```python
from build123d import *

# Parameters (mm, degrees)
SKETCH1_W           = 62
SKETCH1_H           = 42
BOSS_EXTRUDE1_DEPTH = 30
SKETCH2_R           = 10
CUT_EXTRUDE1_DEPTH  = 6
CUT_EXTRUDE2_START  = -2
SKETCH3_W           = 60
SKETCH3_H           = 40
CUT_EXTRUDE2_DEPTH  = 27
CUT_EXTRUDE3_REACH  = 62.547
SKETCH4_W           = 60
SKETCH4_H           = 28
SKETCH5_W           = 20
SKETCH5_H           = 1
CUT_EXTRUDE4_DEPTH  = 27
BOSS_EXTRUDE2_START = 2
BOSS_EXTRUDE2_DEPTH = 5
BOSS_EXTRUDE3_START = -7
BOSS_EXTRUDE3_DEPTH = 5
SKETCH10_W          = 15.255500618
SKETCH10_H          = 40
CUT_EXTRUDE5_DEPTH  = 1


with BuildPart() as part:
    # Sketch1 → Boss-Extrude1 (new body)
    with BuildSketch(Plane.XY):
        with Locations((0.653781513, -2.494957983)):
            Rectangle(SKETCH1_W, SKETCH1_H)
    extrude(amount=BOSS_EXTRUDE1_DEPTH)

    # Sketch2 → Cut-Extrude1 (cut)
    with BuildSketch(Plane.XY.offset(30)):
        with Locations((-15.346218487, -8.494957983)):
            Circle(SKETCH2_R)
    extrude(amount=-CUT_EXTRUDE1_DEPTH, mode=Mode.SUBTRACT)

    # Sketch3 → Cut-Extrude2 (cut)
    with BuildSketch(Plane.XY.offset(30).offset(CUT_EXTRUDE2_START)):
        with Locations((0.653781513, -2.494957983)):
            Rectangle(SKETCH3_W, SKETCH3_H)
    extrude(amount=-CUT_EXTRUDE2_DEPTH, mode=Mode.SUBTRACT)

    # Cut-Extrude3: up to this face of the body (flat: up to its plane)
    cut_extrude3_end = Plane(part.part.faces().sort_by_distance((0.653781513, -22.494957983, 14.5))[0])
    # Sketch4 → Cut-Extrude3 (cut, up to the picked face)
    with BuildSketch(Plane(origin=(0, 18.505042017, 0), x_dir=(1, 0, 0), z_dir=(0, 1, 0)), mode=Mode.PRIVATE) as cut_extrude3_sk1:
        with Locations((0.653781513, -15)):
            Rectangle(SKETCH4_W, SKETCH4_H)
    cut_extrude3_tool1 = split(extrude(cut_extrude3_sk1.sketch, amount=-CUT_EXTRUDE3_REACH, mode=Mode.PRIVATE), bisect_by=cut_extrude3_end, keep=Keep.BOTH, mode=Mode.PRIVATE)
    add(cut_extrude3_tool1.solids().sort_by(Axis((0.653782, 18.505042, 15), (0, -1, 0)))[0], mode=Mode.SUBTRACT)

    # Sketch5 → Cut-Extrude4 (cut)
    with BuildSketch(Plane(origin=(0, 18.505042017, 0), x_dir=(1, 0, 0), z_dir=(0, 1, 0))):
        with Locations((-15.346218487, -29.5)):
            Rectangle(SKETCH5_W, SKETCH5_H)
    extrude(amount=-CUT_EXTRUDE4_DEPTH, mode=Mode.SUBTRACT)

    # Sketch7 → Boss-Extrude2 (add)
    with BuildSketch(Plane(origin=(0, 0, 0), x_dir=(0, 0, -1), z_dir=(1, 0, 0)).offset(BOSS_EXTRUDE2_START)):
        with BuildLine():
            Line((0, 7.999642933), (15, 7.999642933))
            ThreePointArc((15, 7.999642933), (25, -2.000357067), (15, -12.000357067))
            Line((15, -12.000357067), (0, -12.000357067))
            Line((0, -12.000357067), (0, 7.999642933))
        make_face()
    extrude(amount=BOSS_EXTRUDE2_DEPTH)

    # Sketch8 → Boss-Extrude3 (add)
    with BuildSketch(Plane(origin=(0, 0, 0), x_dir=(0, 0, -1), z_dir=(1, 0, 0)).offset(BOSS_EXTRUDE3_START)):
        with BuildLine():
            Line((0, -12.000357067), (0, 7.999642933))
            Line((0, 7.999642933), (15, 7.999642933))
            ThreePointArc((15, 7.999642933), (25, -2.000357067), (15, -12.000357067))
            Line((15, -12.000357067), (0, -12.000357067))
        make_face()
    extrude(amount=BOSS_EXTRUDE3_DEPTH)

    # Sketch10 → Cut-Extrude5 (cut)
    with BuildSketch(Plane.ZY.offset(30.346218487)):
        with Locations((9.627750309, -1.494957983)):
            Rectangle(SKETCH10_W, SKETCH10_H)
    extrude(amount=-CUT_EXTRUDE5_DEPTH, mode=Mode.SUBTRACT)


solid = part.part
```
Input: part model. Units: mm. Frame: model coordinates. A direction names the side the tool comes from. Round coordinates to 2 decimals unless told otherwise and drop trailing zeros. Loops run counter-clockwise (first coordinate to the right, second up) from the corner with the lowest first, then second, coordinate; pieces in that order, holes last. Notation, with made-up numbers: (83.5, 49.25) -> (138.5, 49.25) arc R35 cw to (138.5, 87.25) -> close; hole circle Ø8 at (51.5, -15.5). An arc over 180 degrees is marked (long way). Use one line per item in the form item = value. Start each with the question number.
Item 1: Section query B-B on x = 11. Return the cut outline in (y, z), then the cut area to 3 significant figures.
Item 2: Set-up query: faces 1 (the face through (-5, 8, -7)), 2 (the face through (-29.346, -2, 21)), 3 (the face through (-7, -2, -13)), 4 (the face through (4, -12, -8)). Return all of +Z, -Z, +X, -X, +Y, -Y with unobstructed straight access to the full face (end or side cutting, diameter ignored); none if empty.
Item 3: Section query C-C on y = -5.5. Return the cut outline in (x, z).
Item 4: Mould query, pull axis Z, two halves, no side actions, for faces 5 (the face through (0, -22.495, 15)), 6 (the face through (7, -2, 30)), 7 (the face through (-30, 18.505, 25)). Classes: pulls with the +Z half, pulls with the -Z half, needs draft (parallel to the pull), parting line crosses it, or undercut.
Item 5: Section query D-D on z = 26. Return the cut outline in (x, y).
Item 6: Material intervals for L1, parallel to X at y = 13.5, z = 18.5; L2, parallel to Z at x = 21.5, y = -2; L3, parallel to X at y = 2, z = -12, sorted ascending. Write a range as from..to.
Item 7: Contact query for flat-ended pins moving along their axis: pin 1 Ø4 at (x, y) = (-20.5, -4) entering from +Z; pin 2 Ø8 at (x, y) = (-22, 7) entering from -Z; pin 3 Ø6 at (x, y) = (-12, -17) entering from +Z; pin 4 Ø14 at (x, z) = (-10.5, 18.5) entering from +Y. Output: stop coordinate, or through.
Item 8: Section query A-A on z = -5. Return the cut outline in (x, y), then the cut area to 3 significant figures.
Ans:
q1.outline = (-23.49, 0) -> (18.51, 0) -> (18.51, 1) -> (-22.49, 1) -> (-22.49, 29) -> (18.51, 29) -> (18.51, 30) -> (-23.49, 30) -> close
q1.area = 112 mm^2
q2.face_1 = -Z, +X, -X, +Y
q2.face_2 = +Y
q2.face_3 = -Z, -X, +Y, -Y
q2.face_4 = -Z, +X, -X, -Y
q3.outline = (-30.35, 0) -> (-7, 0) -> (-7, -24.37) -> (-2, -24.37) -> (-2, 0) -> (2, 0) -> (2, -24.37) -> (7, -24.37) -> (7, 0) -> (31.65, 0) -> (31.65, 30) -> (-5.35, 30) -> (-5.35, 29) -> (30.65, 29) -> (30.65, 1) -> (-29.35, 1) -> (-29.35, 2) -> (-30.35, 2) -> close; (-30.35, 17.26) -> (-29.35, 17.26) -> (-29.35, 29) -> (-25.35, 29) -> (-25.35, 30) -> (-30.35, 30) -> close
q4.face_5 = undercut
q4.face_6 = pulls with the +Z half
q4.face_7 = needs draft
q5.outline = (-30.35, -23.49) -> (31.65, -23.49) -> (31.65, 18.51) -> (30.65, 18.51) -> (30.65, -22.49) -> (-29.35, -22.49) -> (-29.35, 18.51) -> (-30.35, 18.51) -> close
q6.L1 = -30.35..-29.35, 30.65..31.65
q6.L2 = 0..1, 29..30
q6.L3 = -7..-2, 2..7
q7.pin_1 = 1
q7.pin_2 = 0
q7.pin_3 = 30
q7.pin_4 = -22.49
q8.outline = (-7, -12) -> (-2, -12) -> (-2, 8) -> (-7, 8) -> close; (2, -12) -> (7, -12) -> (7, 8) -> (2, 8) -> close
q8.area = 200 mm^2
